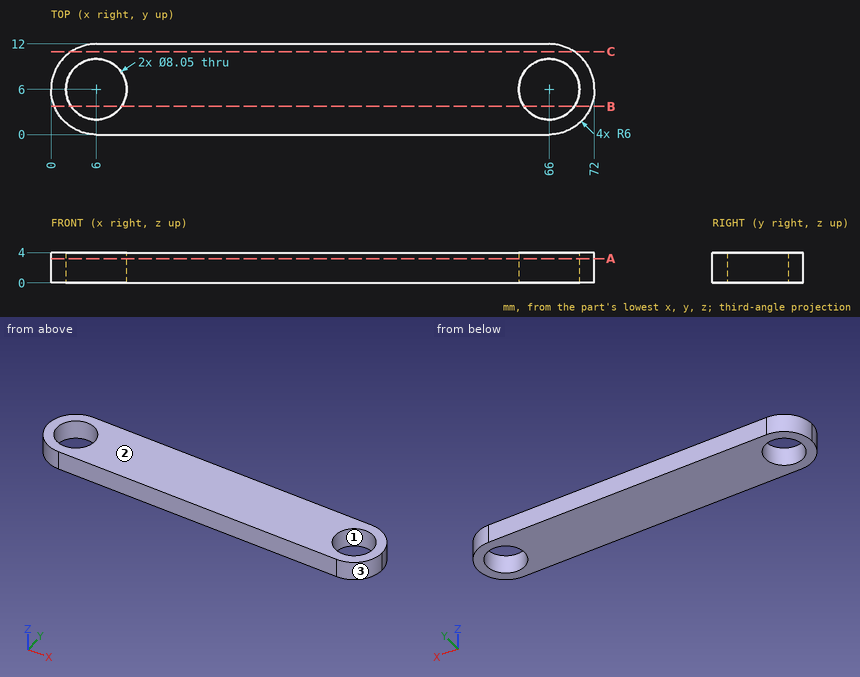
Study the drawing (mm; zero at the part's minimum x, y, z) and answer. Give positions to 0.01 mm unless a question says otherwise; leave off trailing zeros. Write each loop counter-clockwise with the first axis right and the second up, starting at its lowest first coordinate (ties: lowest second). Pieces come first, ordered by that corner, then holes. Notation, with made-up numbers: (46.25, 55.25) -> (89.25, 55.25) arc R22 cw to (89.25, 68.25) -> close; hole circle Ø5 at (55.5, 14.25). An arc over 180 degrees is marked (long way). Answer as a JSON object with one key per item and string values. Group by question number.
1) Find section B-B (y = 3.75). Write down the section's boundary in (x, z), and give its area (3 significant figures).
2) This flat-tipped pin is pushed along its axis until it touches: P1, Ø5, axis at x = 6, y = 6, coming from the -Z side. Where does it stop, or does it pass through?
3) Find section A-A (z = 3.2). Count the separate pieces of the cut face and the enclosed holes in it, and give its area (3 significant figures).
4) Find section C-C (y = 11). Write down the section's boundary in (x, z), and give its area (3 significant figures).
5) Consider L1, parallel to X at y = 6, z = 2.8 (3 decimals); L2, parallel to Y at x = 6, z = 2.4 (3 decimals); L3, parallel to X at y = 4, z = 1.25. Determine where each line is inside the solid, lowest interval first. Write a range as from..to.
6) The mould has two halves that part along Y. Classify the marked faces 1, 2 and 3: +Y half, -Y half, draft (parallel to the pull), parting line (faces both ways), or undercut.
Values follow:
{
 "1": {"outline": "(0.44, 0) -> (2.66, 0) -> (2.66, 4) -> (0.44, 4) -> close; (9.34, 0) -> (62.66, 0) -> (62.66, 4) -> (9.34, 4) -> close; (69.34, 0) -> (71.56, 0) -> (71.56, 4) -> (69.34, 4) -> close", "area": "231 mm2"},
 "2": {"P1": "passes through"},
 "3": {"separate pieces": "1", "enclosed holes": "2", "area": "731 mm2"},
 "4": {"outline": "(2.68, 0) -> (69.32, 0) -> (69.32, 4) -> (2.68, 4) -> close", "area": "267 mm2"},
 "5": {"L1": "x = 0..1.975, 10.025..61.975, 70.025..72", "L2": "y = 0..1.975, 10.025..12", "L3": "x = 0.34..2.51, 9.49..62.51, 69.49..71.66"},
 "6": {"face 1": "undercut", "face 2": "draft", "face 3": "-Y half"}
}
